```python
from build123d import *

# Parameters (mm, degrees)
BOSS_EXTRUDE1_DEPTH = 3
SKETCH2_R           = 1
CUT_EXTRUDE1_DEPTH  = 15.456832295
FILLET1_R           = 1


with BuildPart() as part:
    # Sketch1 → Boss-Extrude1 (new body)
    with BuildSketch(Plane(origin=(0, 0, 0), x_dir=(1, 0, 0), z_dir=(0, 1, 0))):
        with BuildLine():
            Line((-10, 0), (-10, -10))
            Line((-10, -10), (10, -10))
            Line((10, -10), (10, 0))
            ThreePointArc((10, 0), (0, 10), (-10, 0))
        make_face()
    extrude(amount=BOSS_EXTRUDE1_DEPTH)

    # Sketch2 → Cut-Extrude1 (cut, through all)
    with BuildSketch(Plane(origin=(0, 3, 0), x_dir=(1, 0, 0), z_dir=(0, 1, 0))):
        with Locations(Location((0, 0, 0), (0, 0, 270))):
            Circle(SKETCH2_R)
    extrude(amount=-CUT_EXTRUDE1_DEPTH, mode=Mode.SUBTRACT)

    # Fillet1
    fillet1_edges = [part.edges().sort_by_distance(p)[0] for p in [
        (10, 3, 5),
        (0, 3, -10),
        (0, 0, 10),
        (-10, 3, 5),
    ]]
    fillet(fillet1_edges, radius=FILLET1_R)


solid = part.part
```
Source: CAD feature listing. Evaluate the final solid. Frame: model axes, mm. Round coordinates to 2 decimals unless told otherwise and drop trailing zeros. Loops run counter-clockwise (first coordinate to the right, second up) from the corner with the lowest first, then second, coordinate; pieces in that order, holes last.
1. Section query A-A on x = 0. Output: boundary loops of the cut face in (y, z).
2. Mould query, pull axis X, two halves, no side actions, for faces 1 (the cylindrical face through (-1, 2, 0)), 2 (the flat face through (10, 1, 5)), 3 (the cylindrical face through (0.14, 0.301, 9.715)). Classes: released by +X, released by -X, zero draft, split by the parting line, or undercut.
3. Ray query, L1, parallel to X at y = 0.9, z = 0; L2, parallel to X at y = 2.15, z = 6.75; L3, parallel to X at y = 0.1, z = -5.5. Return the intervals inside material, ascending.
4. Section query B-B on y = 1.4. Output: boundary loops of the cut face in (x, z).
5. Contact query for a flat-ended pin moving along its axis: pin 1 (1.5 mm diameter, centred on y = 2, z = -1, fed in from +X). Output: stop coordinate, or through.
6. Section query C-C on y = 2.7. Output: boundary loops of the cut face in (x, z), and give its area (3 significant figures).
Answers below:
1. outline: (0, -10) - (2, -10) arc R1 ccw to (3, -9) - (3, -1) - (0, -1) - close; (0, 1) - (3, 1) - (3, 10) - (1, 10) arc R1 ccw to (0, 9) - close
2. face 1: undercut
2. face 2: released by +X
2. face 3: zero draft
3. L1: x = -10 to -1, 1 to 10
3. L2: x = -9.99 to 9.99
3. L3: x = -8.35 to 8.35
4. outline: (-10, 0) arc R10 ccw to (10, 0) - (10, 10) - (-10, 10) - close; hole circle Ø2 at (0, 0)
5. pin 1: stops at x = 10
6. outline: (-9.71, 0) arc R9.71 ccw to (9.71, 0) - (9.71, 10) - (-9.71, 10) - close; hole circle Ø2 at (0, 0)
6. area: 339 mm2
